For this review, take the finished solid that the model builds, in its own axes (mm). Give positions to 0.01 mm unless a question says otherwise; leave off trailing zeros. Order: outer loops, then holes, each group sorted by start corner. A loop starts at its lowest first (then second) coordinate and runs counter-clockwise, first axis right, second up. Notation, with made-up numbers: (30, 17) -> (59, 17) arc R19 ccw to (59, 23) -> close; hole circle Ø4 at (-8.75, 7). An arc over 180 degrees is marked (long way). Return JSON: item names as keys, results as strings. Group by question number.
1) Add section B-B (z = 0). Give the boundary of the cut face in (x, y).
2) To check wall thickness, follow line 1 along Z through (x, y) = (100, -6); line 2 along X through (y, z) = (-8.5, 2); line 3 along X through (y, z) = (-3.75, 3). State the ranges of each line that lie inside material, in increasing order.
3) Add section A-A (x = 6). Give the boundary of the cut face in (y, z), then the cut area to 3 significant figures.
4) Add section C-C (y = -5). Give the boundary of the cut face in (x, z), then the cut area to 3 significant figures.
5) Add section D-D (x = 100). Give the boundary of the cut face in (y, z).
6) The part is to be moulded in two halves that separate along X. For faces 1 (the face through (74, -10, 0)), 2 (the face through (165, -5, 0)), 3 (the face through (92.507, -4.93, 0.33)), 4 (the face through (-7.493, -4.93, 0.33)), say which applies: released by +X, released by -X, zero draft, split by the parting line, or undercut.
7) Insertion check: P1, Ø12, axis at x = 100, z = 0, coming from the +Y side; P2, Ø1, axis at y = -6.5, z = 4, coming from the -X side. Each pin has a flat end and moves straight along its axis. Give the tip position at first contact, or say it passes through.
from build123d import *

# Parameters (mm, degrees)
F0_R     = 7.5
F1_DEPTH = 10


with BuildPart() as f1:
    # F0 (on Front) → F1 (new body)
    with BuildSketch(Plane.XZ):
        with BuildLine():
            Line((150, 15), (0, 15))
            ThreePointArc((0, 15), (-15, 0), (0, -15))
            Line((0, -15), (150, -15))
            ThreePointArc((150, -15), (165, 0), (150, 15))
        make_face()
        Circle(F0_R, mode=Mode.SUBTRACT)
        with Locations((100, 0)):
            Circle(F0_R, mode=Mode.SUBTRACT)
        with Locations((150, 0)):
            Circle(F0_R, mode=Mode.SUBTRACT)
    extrude(amount=F1_DEPTH)


solid = f1.part
Evaluation:
{
 "1": {"outline": "(-15, -10) -> (-7.5, -10) -> (-7.5, 0) -> (-15, 0) -> close; (7.5, -10) -> (92.5, -10) -> (92.5, 0) -> (7.5, 0) -> close; (107.5, -10) -> (142.5, -10) -> (142.5, 0) -> (107.5, 0) -> close; (157.5, -10) -> (165, -10) -> (165, 0) -> (157.5, 0) -> close"},
 "2": {"line 1": "-15 to -7.5, 7.5 to 15", "line 2": "-14.87 to -7.23, 7.23 to 92.77, 107.23 to 142.77, 157.23 to 164.87", "line 3": "-14.7 to -6.87, 6.87 to 93.13, 106.87 to 143.13, 156.87 to 164.7"},
 "3": {"outline": "(-10, -15) -> (0, -15) -> (0, -4.5) -> (-10, -4.5) -> close; (-10, 4.5) -> (0, 4.5) -> (0, 15) -> (-10, 15) -> close", "area": "210 mm^2"},
 "4": {"outline": "(0, -15) -> (150, -15) arc R15 ccw to (150, 15) -> (0, 15) arc R15 ccw to start; hole circle Ø15 at (0, 0); hole circle Ø15 at (100, 0); hole circle Ø15 at (150, 0)", "area": "4,680 mm^2"},
 "5": {"outline": "(-10, -15) -> (0, -15) -> (0, -7.5) -> (-10, -7.5) -> close; (-10, 7.5) -> (0, 7.5) -> (0, 15) -> (-10, 15) -> close"},
 "6": {"face 1": "zero draft", "face 2": "released by +X", "face 3": "undercut", "face 4": "undercut"},
 "7": {"P1": "through", "P2": "x = -14.59"}
}
